from build123d import *

# Parameters (mm, degrees)
BOSS_EXTRUDE1_DEPTH                                 = 17.78
CBORE_FOR_00_BINDING_HEAD_MACHINE_SCREW_D           = 13.4874
CBORE_FOR_00_BINDING_HEAD_MACHINE_SCREW_CBORE_D     = 23.876
CBORE_FOR_00_BINDING_HEAD_MACHINE_SCREW_CBORE_DEPTH = 1.016
BOSS_EXTRUDE3_DEPTH                                 = 19.05
SKETCH10_R                                          = 12.7
CUT_EXTRUDE1_DEPTH                                  = 19.05
F_29_0_136_DIAMETER_HOLE1_REACH                     = 117.235
F_29_0_136_DIAMETER_HOLE1_BORE_R                    = 1.7272
FILLET1_R                                           = 2.54
FILLET2_R                                           = 2.54
FILLET3_R                                           = 2.54
FILLET4_R                                           = 2.54
FILLET5_START                                       = -22.86
FILLET5_3_DEPTH                                     = 45.72


with BuildPart() as part:
    # Sketch1 → Boss-Extrude1 (new body)
    with BuildSketch(Plane(origin=(0, 0, 0), x_dir=(1, 0, 0), z_dir=(0, 1, 0))):
        with BuildLine():
            Line((63.246, 22.032212417), (10.16, 36.720354029))
            ThreePointArc((10.16, 36.720354029), (0, 38.1), (-10.16, 36.720354029))
            Line((-10.16, 36.720354029), (-63.246, 22.032212417))
            ThreePointArc((-63.246, 22.032212417), (-80.01, 0), (-63.246, -22.032212417))
            Line((-63.246, -22.032212417), (-10.16, -36.720354029))
            ThreePointArc((-10.16, -36.720354029), (0, -38.1), (10.16, -36.720354029))
            Line((10.16, -36.720354029), (63.246, -22.032212417))
            ThreePointArc((63.246, -22.032212417), (80.01, 0), (63.246, 22.032212417))
        make_face()
    extrude(amount=BOSS_EXTRUDE1_DEPTH)

    # CBORE for #00 Binding Head Machine Screw2 (through all)
    with Locations(Plane(origin=(0, 17.78, 0), x_dir=(1, 0, 0), z_dir=(0, 1, 0))):
        with Locations((-57.15, 0), (57.15, 0)):
            CounterBoreHole(CBORE_FOR_00_BINDING_HEAD_MACHINE_SCREW_D / 2, CBORE_FOR_00_BINDING_HEAD_MACHINE_SCREW_CBORE_D / 2, CBORE_FOR_00_BINDING_HEAD_MACHINE_SCREW_CBORE_DEPTH)

    # Sketch7 → Boss-Extrude3 (add, symmetric)
    with BuildSketch(Plane(origin=(0, 0, 0), x_dir=(0, -1, 0), z_dir=(0.7071067811865464, 0, 0.7071067811865488))):
        with BuildLine():
            Line((-48.26, -25.4), (-17.78, -25.4))
            Line((-17.78, -25.4), (-17.78, 25.4))
            Line((-17.78, 25.4), (-48.26, 25.4))
            ThreePointArc((-48.26, 25.4), (-73.66, 0), (-48.26, -25.4))
        make_face()
    extrude(amount=BOSS_EXTRUDE3_DEPTH, both=True)

    # Sketch10 → Cut-Extrude1 (cut, symmetric)
    with BuildSketch(Plane(origin=(0, 0, 0), x_dir=(0, -1, 0), z_dir=(0.7071067811865464, 0, 0.7071067811865488))):
        with Locations(Location((-48.26, 0, 0), (0, 0, 90))):
            Circle(SKETCH10_R)
    extrude(amount=CUT_EXTRUDE1_DEPTH, both=True, mode=Mode.SUBTRACT)

    # #29 (0.136) Diameter Hole1 bore (on position points) → #29 (0.136) Diameter Hole1 (cut, up to next)
    with BuildSketch(Plane.ZX.offset(73.66), mode=Mode.PRIVATE) as f_29_0_136_diameter_hole1_sk1:
        Circle(F_29_0_136_DIAMETER_HOLE1_BORE_R)
    f_29_0_136_diameter_hole1_tool1 = extrude(f_29_0_136_diameter_hole1_sk1.sketch, amount=-F_29_0_136_DIAMETER_HOLE1_REACH, mode=Mode.PRIVATE) & part.part
    add(f_29_0_136_diameter_hole1_tool1.solids().sort_by_distance((0, 73.66, 0))[0], mode=Mode.SUBTRACT)

    # Fillet1
    fillet1_edges = [part.edges().sort_by_distance(p)[0] for p in [
        (-36.703, 17.78, -29.376283223),
        (-80.01, 17.78, 0),
        (-36.703, 17.78, 29.376283223),
        (0, 17.78, 38.1),
        (36.703, 17.78, 29.376283223),
        (80.01, 17.78, 0),
        (36.703, 17.78, -29.376283223),
        (0, 17.78, -38.1),
    ]]
    fillet(fillet1_edges, radius=FILLET1_R)

    # Fillet2
    fillet2_edges = [part.edges().sort_by_distance(p)[0] for p in [
        (31.430896424, 33.02, -4.490128061),
        (-4.490128061, 33.02, 31.430896424),
        (13.470384182, 73.66, 13.470384182),
    ]]
    fillet(fillet2_edges, radius=FILLET2_R)

    # Fillet3
    fillet3_edges = [part.edges().sort_by_distance(p)[0] for p in [
        (17.06248663, 17.78, -18.858537854),
        (13.470384182, 17.78, 13.470384182),
        (-18.858537854, 17.78, 17.06248663),
        (30.378793975, 17.78, -4.490128061),
        (-4.490128061, 17.78, 30.378793975),
    ]]
    fillet(fillet3_edges, radius=FILLET3_R)

    # Fillet4
    # the kernel refuses this fillet: 2.54 mm, written as the material it takes off along each edge
    with BuildSketch(Plane(origin=(-33.226947648, 20.32, 6.286179285), x_dir=(-0.4226145849074772, 0.8017442392976469, 0.42261458490747583), z_dir=(0.5669187883846173, 0.5976672776328292, -0.5669187883846153))) as fillet4_piece_1_section:
        with BuildLine():
            CenterArc((2.54 + FILLET4_R, FILLET4_R), FILLET4_R, 180, 90)
            Line((2.54, FILLET4_R), (2.54, 0))
            Line((2.54, 0), (2.54 + FILLET4_R, 0))
        make_face()
    fillet4_piece_1 = revolve(axis=Axis((-33.226947648, 20.32, 6.286179285), (0.7071067811865464, 0, 0.7071067811865488)), revolution_arc=233.296989237, mode=Mode.PRIVATE)
    fillet4_piece_1 = split(fillet4_piece_1, bisect_by=Plane(origin=(-33.226947648, 17.78, 6.286179285), z_dir=(0, 1, 0)), keep=Keep.TOP, mode=Mode.PRIVATE)
    add(fillet4_piece_1, mode=Mode.SUBTRACT)
    with BuildSketch(Plane(origin=(6.286179285, 20.32, -33.226947648), x_dir=(0.4226145849074753, 0.8017442392976486, -0.42261458490747456), z_dir=(-0.5669187883846184, 0.597667277632827, 0.5669187883846165))) as fillet4_piece_2_section:
        with BuildLine():
            CenterArc((2.54 + FILLET4_R, -FILLET4_R), FILLET4_R, 90, 90)
            Line((2.54, -FILLET4_R), (2.54, 0))
            Line((2.54, 0), (2.54 + FILLET4_R, 0))
        make_face()
    fillet4_piece_2 = revolve(axis=Axis((6.286179285, 20.32, -33.226947648), (-0.7071067811865464, 0, -0.7071067811865488)), revolution_arc=233.296989237, mode=Mode.PRIVATE)
    fillet4_piece_2 = split(fillet4_piece_2, bisect_by=Plane(origin=(6.286179285, 17.78, -33.226947648), z_dir=(0, 1, 0)), keep=Keep.TOP, mode=Mode.PRIVATE)
    add(fillet4_piece_2, mode=Mode.SUBTRACT)
    with BuildSketch(Plane(origin=(-31.430896424, 48.26, 4.490128061), x_dir=(0.7071067811865488, 0, -0.7071067811865462), z_dir=(0, -1, 0)), Plane(origin=(4.490128061, 20.32, -31.430896424), x_dir=(-0.707106781186549, 0, 0.7071067811865461), z_dir=(0, 1, 0))) as fillet4_piece_3:
        with BuildLine():
            CenterArc((FILLET4_R, FILLET4_R), FILLET4_R, 180, 90)
            Line((0, FILLET4_R), (0, 0))
            Line((0, 0), (FILLET4_R, 0))
        make_face()
    extrude(amount=27.94, mode=Mode.SUBTRACT)
    with BuildSketch(Plane(origin=(-13.470384182, 48.26, -13.470384182), x_dir=(0.7071067811865487, 0, -0.7071067811865464), z_dir=(0, -1, 0))) as fillet4_piece_4:
        with BuildLine():
            CenterArc((25.4 - FILLET4_R, FILLET4_R), FILLET4_R, 270, 90)
            Line((25.4, FILLET4_R), (25.4, 0))
            Line((25.4, 0), (25.4 - FILLET4_R, 0))
        make_face()
    revolve(axis=Axis((-13.470384182, 48.26, -13.470384182), (0.7071067811865464, 0, 0.7071067811865488)), revolution_arc=180, mode=Mode.SUBTRACT)

    # Fillet5: read off the stored shape, not the designer's step
    # Fillet5 outline → Fillet5 (revolve)
    with BuildSketch(Plane(origin=(-27.838793975, 0, 4.490128061), x_dir=(1, 0, 0), z_dir=(0, 0, 1))):
        with BuildLine():
            ThreePointArc((5.08, 17.78), (3.283948776, 18.523948776), (2.54, 20.32))
            Line((2.54, 20.32), (2.54, 17.78))
            Line((2.54, 17.78), (5.08, 17.78))
        make_face()
    revolve(axis=Axis((-27.838793975, 0, 4.490128061), (0, 1, 0)))

    # Fillet5 2 outline → Fillet5 2 (revolve)
    with BuildSketch(Plane(origin=(4.490128061, 0, -27.838793975), x_dir=(1, 0, 0), z_dir=(0, 0, 1))):
        with BuildLine():
            ThreePointArc((5.08, 17.78), (3.283948776, 18.523948776), (2.54, 20.32))
            Line((2.54, 20.32), (2.54, 17.78))
            Line((2.54, 17.78), (5.08, 17.78))
        make_face()
    revolve(axis=Axis((4.490128061, 0, -27.838793975), (0, 1, 0)))

    # Fillet5 3 outline → Fillet5 3 (add)
    with BuildSketch(Plane(origin=(0, 0, 0), x_dir=(0.707106781186546, 0, 0.707106781186549), z_dir=(0.707106781186549, 0, -0.707106781186546)).offset(FILLET5_START)):
        with BuildLine():
            ThreePointArc((-21.59, -17.78), (-19.793948776, -18.523948776), (-19.05, -20.32))
            Line((-19.05, -20.32), (-19.05, -17.78))
            Line((-19.05, -17.78), (-21.59, -17.78))
        make_face()
    extrude(amount=FILLET5_3_DEPTH)


solid = part.part
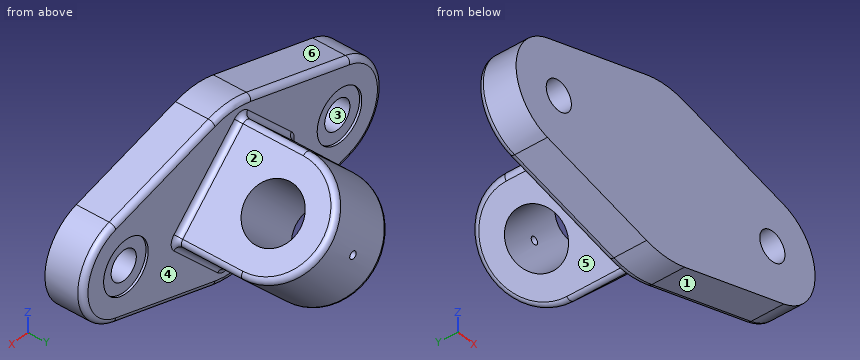
Check sheet for the modelled part. Datum: model origin and axes. Units: mm. Face numbers are marked on the shaded views. A direction names the side the tool comes from. Give positions to 0.01 mm unless a question says otherwise; leave off trailing zeros. Order: outer loops, then holes, each group sorted by start corner. A loop starts at its lowest first (then second) coordinate and runs counter-clockwise, first axis right, second up. Notation, with made-up numbers: (10, 75) - (62, 75) arc R13 cw to (62, 81) - close; hole circle Ø11 at (6, -34.5). An arc over 180 degrees is marked (long way). Answer as CSV lines item,"result".
1. Go/stop test with flat-tipped pins: P1, Ø5, axis at y = 24, z = 1.5, coming from the -X side; P2, Ø10, axis at x = -15.5, y = 59, coming from the -Z side; P3, Ø4, axis at x = 47, z = -5.5, coming from the +Y side. Record where each tip stops, or that it passes through.
Result sheet:
P1,"x = -30.33"
P2,"z = -16.26"
P3,"y = 17.78"
2. Mould release check, pull along Z, two halves, no side actions. Record for the marked faces 1, 2 and 3: released by +Z, released by -Z, zero draft, split by the parting line, or undercut.
Result sheet:
face 1,"released by -Z"
face 2,"released by +Z"
face 3,"undercut"
3. Tool access check on the marked faces 4, 5 and 6. Record the directions out of +Z, -Z, +X, -X, +Y, -Y that give a thin tool (end or side, any length) a straight path to the whole face; none if there is none.
Result sheet:
face 4,"+Y"
face 5,"-Z, -X, +Y"
face 6,"+Z, -X, +Y, -Y"
4. Scan lines: probe 1 along X at (y, z) = (10.5, -5); probe 2 along Z at (x, y) = (-57.15, 17.4); probe 3 along Z at (x, y) = (-57.15, 17.2). Record each from-to range of solid material in increasing order. Write a range as from..to.
Result sheet:
probe 1,"-79.46..-61.68, -52.62..52.62, 61.68..79.46"
probe 2,"-22.47..-11.94, 11.94..22.47"
probe 3,"-22.76..-11.94, 11.94..22.76"
5. Section check A-A (y = 24). Record the boundary of the cut face in (x, z), then the cut area to 3 significant figures.
Result sheet:
outline,"(-29.63, 2.69) - (2.69, -29.63) arc R2.54 ccw to (6.29, -29.63) - (29.63, -6.29) arc R2.54 ccw to (29.63, -2.69) - (-2.69, 29.63) arc R2.54 ccw to (-6.29, 29.63) - (-29.63, 6.29) arc R2.54 ccw to start"
area,"1,930 mm²"
